Here's the drawing with two shaded views (mm, measured from the low corner). I have some questions. Coordinates: 2 decimals unless noted, no trailing zeros. Write each loop counter-clockwise with the first axis right and the second up, starting at its lowest first coordinate (ties: lowest second). Pieces come first, ordered by that corner, then holes. Notation, with made-up numbers: (-18, -30) -> (1, -30) arc R18 cw to (1, 1) -> close; hole circle Ø9 at (29, 47). An arc over 180 degrees is marked (long way). Put each result on its own line as item: value.
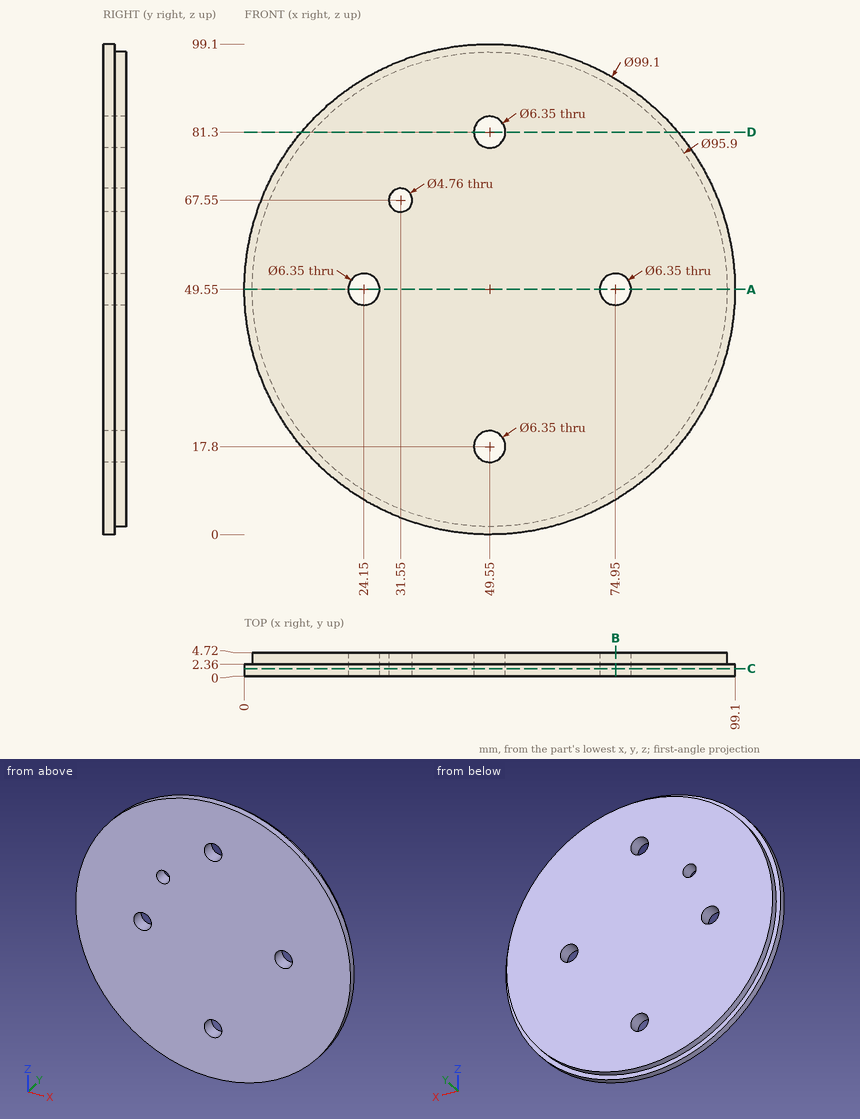
Item 1: Imagine slicing it at C-C on y = 1.5. Write out the boundary of the cut face in (x, z) (3 decimals), then the cut area to 3 significant figures.
Output:
outline: circle Ø99.1 at (49.55, 49.55); hole circle Ø6.35 at (24.15, 49.55); hole circle Ø4.76 at (31.55, 67.55); hole circle Ø6.35 at (49.55, 17.8); hole circle Ø6.35 at (49.55, 81.3); hole circle Ø6.35 at (74.95, 49.55)
area: 7,570 mm²
Item 2: Please list where these lines run through material, in increasing order: line 1 along Z through (x, y) = (49.55, 2.05) (3 decimals); line 2 along Z through (x, y) = (49.55, 2.4) (3 decimals); line 3 along X through (y, z) = (4.05, 52). Write a range as from..to.
Output:
line 1: z = 0..14.625, 20.975..78.125, 84.475..99.1
line 2: z = 1.6..14.625, 20.975..78.125, 84.475..97.5
line 3: x = 1.66..22.13, 26.17..72.93, 76.97..97.44
Item 3: For P1, Ø1, axis at y = 2.5, z = 47.5, coming from the +X side; P2, Ø1.5, axis at x = 11.5, y = 1.5, coming from the +Z side, each with a flat end and sliding along its axis, tell me the tip position at first contact or that it passes through.
Output:
P1: stops at x = 99.08
P2: stops at z = 82.17
Item 4: Imagine slicing it at A-A on z = 49.55. Write out the boundary of the cut face in (x, y) (3 decimals).
Output:
outline: (0, 0) -> (20.975, 0) -> (20.975, 4.72) -> (1.6, 4.72) -> (1.6, 2.36) -> (0, 2.36) -> close; (27.325, 0) -> (71.775, 0) -> (71.775, 4.72) -> (27.325, 4.72) -> close; (78.125, 0) -> (99.1, 0) -> (99.1, 2.36) -> (97.5, 2.36) -> (97.5, 4.72) -> (78.125, 4.72) -> close
Item 5: Imagine slicing it at B-B on x = 75. Write out the boundary of the cut face in (y, z), then the cut area to 3 significant figures.
Output:
outline: (0, 7.04) -> (2.36, 7.04) -> (2.36, 8.91) -> (4.72, 8.91) -> (4.72, 46.38) -> (0, 46.38) -> close; (0, 52.72) -> (4.72, 52.72) -> (4.72, 90.19) -> (2.36, 90.19) -> (2.36, 92.06) -> (0, 92.06) -> close
area: 363 mm²
Item 6: Imagine slicing it at D-D on z = 81.3. Write out the boundary of the cut face in (x, y) (3 decimals), then the cut area to 3 significant figures.
Output:
outline: (11.509, 0) -> (46.375, 0) -> (46.375, 4.72) -> (13.618, 4.72) -> (13.618, 2.36) -> (11.509, 2.36) -> close; (52.725, 0) -> (87.591, 0) -> (87.591, 2.36) -> (85.482, 2.36) -> (85.482, 4.72) -> (52.725, 4.72) -> close
area: 319 mm²
